Work out the finished part from the listing and answer in its coordinate system (mm). Coordinates: 2 decimals unless noted, no trailing zeros. Write each loop counter-clockwise with the first axis right and the second up, starting at its lowest first coordinate (ties: lowest second). Pieces come first, ordered by that corner, then holes. Notation, with made-up numbers: (18, 14) - (50, 14) arc R22 ccw to (50, 27) - close; hole circle Ø6 at (37, -27). An arc over 180 degrees is marked (long way). One line per item, written item: value.
```python
from build123d import *

# Parameters (mm, degrees)
SKETCH1_W           = 33.53
SKETCH1_H           = 12
SKETCH1_R           = 1.5875
BOSS_EXTRUDE1_DEPTH = 0.79375
FILLET1_R           = 4


with BuildPart() as part:
    # Sketch1 → Boss-Extrude1 (new, symmetric)
    with BuildSketch(Plane(origin=(0, 0, 0), x_dir=(1, 0, 0), z_dir=(0, 1, 0))):
        Rectangle(SKETCH1_W, SKETCH1_H)
        with Locations(Location((-10.765, 0, 0), (0, 0, 270))):
            Circle(SKETCH1_R, mode=Mode.SUBTRACT)
        with Locations(Location((10.765, 0, 0), (0, 0, 270))):
            Circle(SKETCH1_R, mode=Mode.SUBTRACT)
    extrude(amount=BOSS_EXTRUDE1_DEPTH, both=True)

    # Fillet1
    fillet1_edges = [part.edges().sort_by_distance(p)[0] for p in [
        (-16.765, 0, -6),
        (16.765, 0, -6),
        (16.765, 0, 6),
        (-16.765, 0, 6),
    ]]
    fillet(fillet1_edges, radius=FILLET1_R)


solid = part.part
```
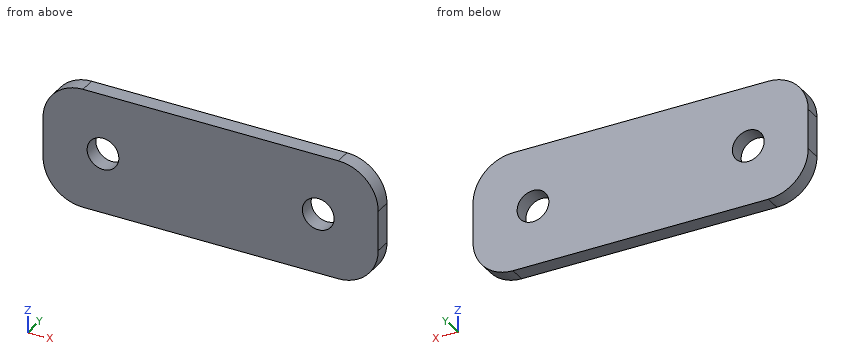
Item 1: Section A-A, the plane z = 0 is taken. Determine the outline of the cut face in (x, y) (1 decimal).
Evaluation:
outline: (-16.8, -0.8) - (-12.4, -0.8) - (-12.4, 0.8) - (-16.8, 0.8) - close; (-9.2, -0.8) - (9.2, -0.8) - (9.2, 0.8) - (-9.2, 0.8) - close; (12.4, -0.8) - (16.8, -0.8) - (16.8, 0.8) - (12.4, 0.8) - close
Item 2: Section B-B, the plane y = 0.1 is taken. Determine the outline of the cut face in (x, z) (1 decimal).
Evaluation:
outline: (-16.8, -2) arc R4 ccw to (-12.8, -6) - (12.8, -6) arc R4 ccw to (16.8, -2) - (16.8, 2) arc R4 ccw to (12.8, 6) - (-12.8, 6) arc R4 ccw to (-16.8, 2) - close; hole circle Ø3.2 at (-10.8, 0); hole circle Ø3.2 at (10.8, 0)
Item 3: Section C-C, the plane x = -12 is taken. Determine the outline of the cut face in (y, z), then the cut area to 3 significant figures.
Evaluation:
outline: (-0.79, -6) - (0.79, -6) - (0.79, -1) - (-0.79, -1) - close; (-0.79, 1) - (0.79, 1) - (0.79, 6) - (-0.79, 6) - close
area: 15.9 mm2
Item 4: Section D-D, the plane z = -1.25 is taken. Determine the outline of the cut face in (x, y) (3 decimals), then the cut area to 3 significant figures.
Evaluation:
outline: (-16.765, -0.794) - (-11.744, -0.794) - (-11.744, 0.794) - (-16.765, 0.794) - close; (-9.786, -0.794) - (9.786, -0.794) - (9.786, 0.794) - (-9.786, 0.794) - close; (11.744, -0.794) - (16.765, -0.794) - (16.765, 0.794) - (11.744, 0.794) - close
area: 47.0 mm2
Item 5: Consider probe 1 along X at (y, z) = (0.4, 0) (1 decimal); probe 2 along X at (y, z) = (0, 1) (3 decimals); probe 3 along Z at (x, y) = (-11.5, 0.1). Determine where each line is inside the solid, lowest interval first.
Evaluation:
probe 1: x = -16.8 to -12.4, -9.2 to 9.2, 12.4 to 16.8
probe 2: x = -16.765 to -11.998, -9.532 to 9.532, 11.998 to 16.765
probe 3: z = -6 to -1.41, 1.41 to 6
